Check sheet for the modelled part. Datum: model origin and axes. Units: mm. Face numbers are marked on the shaded views. Coordinates: 2 decimals unless noted, no trailing zeros. Loops run counter-clockwise (first coordinate to the right, second up) from the corner with the lowest first, then second, coordinate; pieces in that order, holes last. Notation, with made-up numbers: (-10.75, 63) - (39.25, 63) arc R23 ccw to (39.25, 82) - close; hole circle Ø5 at (12, 58.25). An arc over 180 degrees is marked (long way). Use a Markdown table: item, result. Add a question column.
1) Sectioned sample at C-C, the plane y = 2.5. Enter the section's corners in (x, z).
2) Thickness scan on line 1 (Z direction, x = 0, y = 5.75); line 2 (Z direction, x = 4, y = 6); line 3 (X direction, y = 6, z = 11.5). Record the ranges inside material, lowest first.
3) Draft check along X on the marked faces 1, 2, 3 and 4. Enter one of: pulls with the +X half, pulls with the -X half, needs draft (parallel to the pull), parting line crosses it, or undercut.
4) Go/stop test with flat-tipped pins: P1, Ø7.5, axis at x = 0, z = 0, coming from the -Y side; P2, Ø0.5, axis at y = 6.5, z = 4, coming from the -X side; P3, Ø8, axis at x = 1, z = 5, coming from the +Y side. Record where each tip stops, or that it passes through.
5) Sectioned sample at B-B, the plane z = 0. Enter the section's corners in (x, y).
6) Sectioned sample at A-A, the plane x = 0. Enter the section's corners in (y, z).
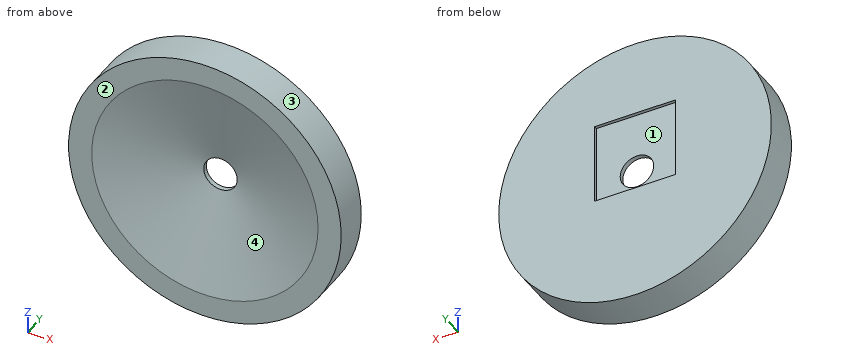
from build123d import *

# Parameters (mm, degrees)
SKETCH5_W          = 15.748
SKETCH5_H          = 15.748
CUT_EXTRUDE1_DEPTH = 6.35


with BuildPart() as part:
    # Sketch3 → Revolve1 (revolve)
    with BuildSketch(Plane.XY):
        Polygon((22, 0), (3.25, 5.442857143), (3.25, 7), (26.5, 7), (26.5, 0), align=None)
    revolve(axis=Axis((0, 0, 0), (0, -1, 0)))

    # Sketch5 → Cut-Extrude1 (cut)
    with BuildSketch(Plane(origin=(0, 12.7, 0), x_dir=(1, 0, 0), z_dir=(0, 1, 0))):
        with Locations((0, -3.964)):
            Rectangle(SKETCH5_W, SKETCH5_H)
    extrude(amount=-CUT_EXTRUDE1_DEPTH, mode=Mode.SUBTRACT)


solid = part.part
Solved:
| question | item | result |
|---|---|---|
| 1 | outline | circle Ø53 at (0, 0); hole circle Ø26.78 at (0, 0) |
| 2 | line 1 | z = -26.5 to -3.25, 3.25 to 26.5 |
| 2 | line 2 | z = -26.2 to 26.2 |
| 2 | line 3 | x = -23.87 to 23.87 |
| 3 | face 1 | undercut |
| 3 | face 2 | needs draft |
| 3 | face 3 | parting line crosses it |
| 3 | face 4 | undercut |
| 4 | P1 | stops at y = 5.3 |
| 4 | P2 | stops at x = -26.23 |
| 4 | P3 | stops at y = 6.35 |
| 5 | outline | (-26.5, 0) - (-22, 0) - (-3.25, 5.44) - (-3.25, 6.35) - (-7.87, 6.35) - (-7.87, 7) - (-26.5, 7) - close; (3.25, 5.44) - (22, 0) - (26.5, 0) - (26.5, 7) - (7.87, 7) - (7.87, 6.35) - (3.25, 6.35) - close |
| 6 | outline | (0, -26.5) - (7, -26.5) - (7, -3.91) - (6.35, -3.91) - (6.35, -3.25) - (5.44, -3.25) - (0, -22) - close; (0, 22) - (5.44, 3.25) - (6.35, 3.25) - (6.35, 11.84) - (7, 11.84) - (7, 26.5) - (0, 26.5) - close |
